Verification items for the finished model (mm, model axes). A direction names the side the tool comes from. Round coordinates to 2 decimals unless told otherwise and drop trailing zeros. Write each loop counter-clockwise with the first axis right and the second up, starting at its lowest first coordinate (ties: lowest second). Pieces come first, ordered by that corner, then holes.
from build123d import *

# Parameters (mm, degrees)
SKETCH_1_R      = 2.55
EXTRUDE_1_DEPTH = 68


with BuildPart() as part:
    # 草图1 → 凸台-拉伸1 (new body)
    with BuildSketch(Plane.XY):
        with BuildLine():
            Line((-3.9, 2.839339828), (-6.560660172, 5.5))
            Line((-6.560660172, 5.5), (-8.2, 5.5))
            Line((-8.2, 5.5), (-8.2, 3.1))
            Line((-8.2, 3.1), (-9.45, 3.1))
            Line((-9.45, 3.1), (-9.45, 3.65))
            Line((-9.45, 3.65), (-10, 3.65))
            Line((-10, 3.65), (-10, 8.5))
            ThreePointArc((-10, 8.5), (-9.560660172, 9.560660172), (-8.5, 10))
            Line((-8.5, 10), (-3.65, 10))
            Line((-3.65, 10), (-3.65, 9.45))
            Line((-3.65, 9.45), (-3.1, 9.45))
            Line((-3.1, 9.45), (-3.1, 8.2))
            Line((-3.1, 8.2), (-5.5, 8.2))
            Line((-5.5, 8.2), (-5.5, 6.560660172))
            Line((-5.5, 6.560660172), (-2.839339828, 3.9))
            Line((-2.839339828, 3.9), (2.839339828, 3.9))
            Line((2.839339828, 3.9), (5.5, 6.560660172))
            Line((5.5, 6.560660172), (5.5, 8.2))
            Line((5.5, 8.2), (3.1, 8.2))
            Line((3.1, 8.2), (3.1, 9.45))
            Line((3.1, 9.45), (3.65, 9.45))
            Line((3.65, 9.45), (3.65, 10))
            Line((3.65, 10), (8.5, 10))
            ThreePointArc((8.5, 10), (9.560660172, 9.560660172), (10, 8.5))
            Line((10, 8.5), (10, 3.65))
            Line((10, 3.65), (9.45, 3.65))
            Line((9.45, 3.65), (9.45, 3.1))
            Line((9.45, 3.1), (8.2, 3.1))
            Line((8.2, 3.1), (8.2, 5.5))
            Line((8.2, 5.5), (6.560660172, 5.5))
            Line((6.560660172, 5.5), (3.9, 2.839339828))
            Line((3.9, 2.839339828), (3.9, -2.839339828))
            Line((3.9, -2.839339828), (6.560660172, -5.5))
            Line((6.560660172, -5.5), (8.2, -5.5))
            Line((8.2, -5.5), (8.2, -3.1))
            Line((8.2, -3.1), (9.45, -3.1))
            Line((9.45, -3.1), (9.45, -3.65))
            Line((9.45, -3.65), (10, -3.65))
            Line((10, -3.65), (10, -8.5))
            ThreePointArc((10, -8.5), (9.560660172, -9.560660172), (8.5, -10))
            Line((8.5, -10), (3.65, -10))
            Line((3.65, -10), (3.65, -9.45))
            Line((3.65, -9.45), (3.1, -9.45))
            Line((3.1, -9.45), (3.1, -8.2))
            Line((3.1, -8.2), (5.5, -8.2))
            Line((5.5, -8.2), (5.5, -6.560660172))
            Line((5.5, -6.560660172), (2.839339828, -3.9))
            Line((2.839339828, -3.9), (-2.839339828, -3.9))
            Line((-2.839339828, -3.9), (-5.5, -6.560660172))
            Line((-5.5, -6.560660172), (-5.5, -8.2))
            Line((-5.5, -8.2), (-3.1, -8.2))
            Line((-3.1, -8.2), (-3.1, -9.45))
            Line((-3.1, -9.45), (-3.65, -9.45))
            Line((-3.65, -9.45), (-3.65, -10))
            Line((-3.65, -10), (-8.5, -10))
            ThreePointArc((-8.5, -10), (-9.560660172, -9.560660172), (-10, -8.5))
            Line((-10, -8.5), (-10, -3.65))
            Line((-10, -3.65), (-9.45, -3.65))
            Line((-9.45, -3.65), (-9.45, -3.1))
            Line((-9.45, -3.1), (-8.2, -3.1))
            Line((-8.2, -3.1), (-8.2, -5.5))
            Line((-8.2, -5.5), (-6.560660172, -5.5))
            Line((-6.560660172, -5.5), (-3.9, -2.839339828))
            Line((-3.9, -2.839339828), (-3.9, 2.839339828))
        make_face()
        Circle(SKETCH_1_R, mode=Mode.SUBTRACT)
    extrude(amount=EXTRUDE_1_DEPTH)


solid = part.part
Q1. Depth check by flat-ended pin: P1, Ø3, axis at x = -0.5, z = 25.5, coming from the -Y side. Enter the tip coordinate at first touch or a pass-through.
Recorded:
P1: stops at y = -3.9
Q2. Sectioned sample at A-A (y = 0). Enter the section's corners in (x, z), plus the area to 3 significant figures.
Recorded:
outline: (-3.9, 0) - (-2.55, 0) - (-2.55, 68) - (-3.9, 68) - close; (2.55, 0) - (3.9, 0) - (3.9, 68) - (2.55, 68) - close
area: 184 mm2
Q3. Material ranges on line 1 along Y through (x, z) = (-7.5, 61); line 2 along Y through (x, z) = (0, 38); line 3 along Y through (x, z) = (-5, 40), recorded low to high.
Recorded:
line 1: y = -10 to -5.5, 5.5 to 10
line 2: y = -3.9 to -2.55, 2.55 to 3.9
line 3: y = -10 to -8.2, -6.06 to -3.94, 3.94 to 6.06, 8.2 to 10
Q4. Sectioned sample at C-C (x = -4.75). Enter the section's corners in (y, z), plus the area to 3 significant figures.
Recorded:
outline: (-10, 0) - (-8.2, 0) - (-8.2, 68) - (-10, 68) - close; (-5.81, 0) - (-3.69, 0) - (-3.69, 68) - (-5.81, 68) - close; (3.69, 0) - (5.81, 0) - (5.81, 68) - (3.69, 68) - close; (8.2, 0) - (10, 0) - (10, 68) - (8.2, 68) - close
area: 533 mm2
Q5. Release check for a two-part mould opening along X. For faces 1 (the cylindrical face through (9.57, -9.55, 33.52)), 2 (the flat face through (3.1, -9, 34)), 3 (the flat face through (-9, -3.1, 34)) record: released by +X, released by -X, zero draft, split by the parting line, or undercut.
Recorded:
face 1: released by +X
face 2: undercut
face 3: zero draft
Q6. Tool access check on faces 4 (the flat face through (9, 3.1, 34)), 5 (the flat face through (-3.9, 0, 34)), 6 (the cylindrical face through (-9.55, -9.57, 33.52)), 7 (the flat face through (4, 8.2, 34)). Record the directions out of +Z, -Z, +X, -X, +Y, -Y that give a thin tool (end or side, any length) a straight path to the whole face; none if there is none.
Recorded:
face 4: +Z, -Z, +X
face 5: +Z, -Z, -X
face 6: +Z, -Z, -X, -Y
face 7: +Z, -Z
